```python
from build123d import *

# Parameters (mm, degrees)
SKETCH2_R           = 2.875
BOSS_EXTRUDE1_DEPTH = 0.71892557
BOSS_EXTRUDE2_START = 1.218925567
SKETCH3_R           = 2.875
BOSS_EXTRUDE2_DEPTH = 1.218925567
SKETCH4_R           = 1.75
CUT_EXTRUDE1_DEPTH  = 14.12440475
FILLET1_R           = 2.5


with BuildPart() as part:
    # Sketch1 → Revolve1 (revolve)
    with BuildSketch(Plane(origin=(0, 0, 0), x_dir=(1, 0, 0), z_dir=(0, 1, 0))):
        with BuildLine():
            Line((8.875, 0.281074433), (6, 0.281074433))
            Line((6, 0.281074433), (6, -5.281074433))
            Line((6, -5.281074433), (8.875, -5.281074433))
            ThreePointArc((8.875, -5.281074433), (10, -2.5), (8.875, 0.281074433))
        make_face()
    revolve(axis=Axis((6, 0, -0.281074433), (0, 0, 1)))

    # Sketch2 → Boss-Extrude1 (add)
    with BuildSketch(Plane(origin=(0, 0, -0.281074433), x_dir=(-1, 0, 0), z_dir=(0, 0, -1))):
        with Locations(Location((-6, 0, 0), (0, 0, 180))):
            Circle(SKETCH2_R)
    extrude(amount=BOSS_EXTRUDE1_DEPTH)

    # Sketch3 → Boss-Extrude2 (add)
    with BuildSketch(Plane.XY.offset(5.281074433).offset(BOSS_EXTRUDE2_START)):
        with Locations((6, 0)):
            Circle(SKETCH3_R)
    extrude(amount=-BOSS_EXTRUDE2_DEPTH)

    # Sketch4 → Cut-Extrude1 (cut, through all)
    with BuildSketch(Plane(origin=(0, 0, -1.000000003), x_dir=(-1, 0, 0), z_dir=(0, 0, -1))):
        with Locations(Location((-6, 0, 0), (0, 0, 180))):
            Circle(SKETCH4_R)
    extrude(amount=-CUT_EXTRUDE1_DEPTH, mode=Mode.SUBTRACT)

    # Fillet1
    # the kernel refuses this fillet: 2.5 mm, written as the material it adds along each edge
    with BuildSketch(Plane(origin=(6, 0, 5.281074433), x_dir=(1, 0, 0), z_dir=(0, -1, 0))) as fillet1_piece_1:
        with BuildLine():
            CenterArc((5.375, 0.873973447), FILLET1_R, 180, 34.216051131)
            Line((2.875, 0.873973447), (2.825, 0.873973447))
            Line((2.825, 0.873973447), (2.825, 0))
            Line((2.825, 0), (2.8390625, -0.03476343))
            ThreePointArc((2.8390625, -0.03476343), (3.063976775, -0.288175252), (3.266346154, -0.559929952))
            Line((3.266346154, -0.559929952), (3.307692308, -0.531814199))
        make_face()
    revolve(axis=Axis((6, 0, 5.281074433), (0, 0, 1)))
    with BuildSketch(Plane(origin=(6, 0, -0.281074433), x_dir=(1, 0, 0), z_dir=(0, -1, 0))) as fillet1_piece_2:
        with BuildLine():
            CenterArc((5.369690775, -0.881768859), FILLET1_R, 145.700811221, 30.56445132)
            Line((2.875, -0.71892557), (2.825106184, -0.715668704))
            ThreePointArc((2.825106184, -0.715668704), (2.825, -0.359462785), (2.825, 0))
            Line((2.825, 0), (2.8390625, 0.03476343))
            ThreePointArc((2.8390625, 0.03476343), (3.062167338, 0.285952954), (3.263119779, 0.55519274))
            Line((3.263119779, 0.55519274), (3.304425092, 0.527017022))
        make_face()
    revolve(axis=Axis((6, 0, -0.281074433), (0, 0, 1)))


solid = part.part
```
Check sheet for the modelled part. Datum: model origin and axes. Units: mm. Round coordinates to 2 decimals unless told otherwise and drop trailing zeros. Order: outer loops, then holes, each group sorted by start corner. A loop starts at its lowest first (then second) coordinate and runs counter-clockwise, first axis right, second up. Notation, with made-up numbers: (-2.5, 18) - (19.5, 18) arc R21 cw to (19.5, 36) - close; hole circle Ø8 at (-11.75, 53). An arc over 180 degrees is marked (long way). Answer as CSV lines item,"result". Start each with the question number.
1) Depth check by flat-ended pin: pin 1 (3 mm diameter, centred on x = 6, y = 0, fed in from +Z); pin 2 (4 mm diameter, centred on x = 9, z = 0.5, fed in from +Y); pin 3 (2 mm diameter, centred on x = 4.5, y = 0.5, fed in from -Z). Enter the tip coordinate at first touch or a pass-through.
2) Scan lines: probe 1 along X at (y, z) = (-1.25, 2.5); probe 2 along Y at (x, z) = (6, 1.25); probe 3 along Y at (x, z) = (6, 2.5). Record each from-to range of solid material in increasing order.
3) Section check A-A (x = 6). Record the cut outline in (y, z) (3 decimals).
4) Section check B-B (z = 2.5). Record the cut outline in (x, y).
5) Draft check along X on faces 1 (the face through (8, 0, 6.5)), 2 (the face through (8.742, 0.864, 6.33)), 3 (the face through (4.25, -0.08, 2.7)). Enter one of: +X half, -X half, draft (parallel to the pull), parting line (faces both ways), or undercut.
Determined:
1,pin 1,"through"
1,pin 2,"y = 3.66"
1,pin 3,"z = -1"
2,probe 1,"2.2 to 4.78, 7.22 to 9.8"
2,probe 2,"-3.8 to -1.75, 1.75 to 3.8"
2,probe 3,"-4 to -1.75, 1.75 to 4"
3,outline,"(-3.308, 4.749) arc R4 ccw to (-3.304, 0.246) arc R2.5 cw to (-2.875, -1) - (-1.75, -1) - (-1.75, 6.5) - (-2.875, 6.5) - (-2.875, 6.155) arc R2.5 cw to start; (1.75, -1) - (2.875, -1) arc R2.5 cw to (3.304, 0.246) arc R4 ccw to (3.308, 4.749) arc R2.5 cw to (2.875, 6.155) - (2.875, 6.5) - (1.75, 6.5) - close"
4,outline,"circle Ø8 at (6, 0); hole circle Ø3.5 at (6, 0)"
5,face 1,"draft"
5,face 2,"parting line"
5,face 3,"undercut"
